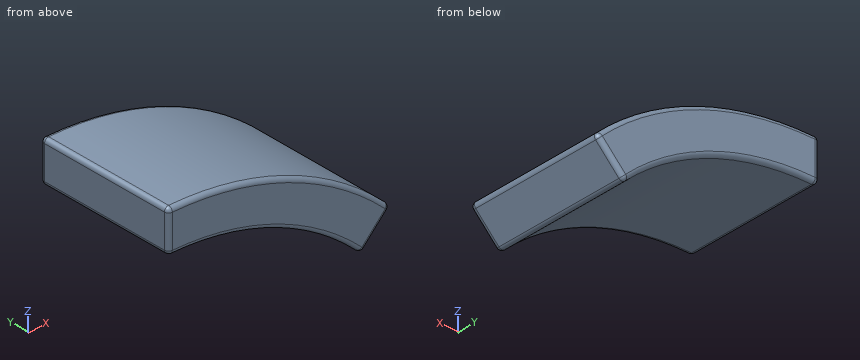
```python
from build123d import *

# Parameters (mm, degrees)
BOSS_EXTRUDE1_DEPTH = 10
FILLET1_R           = 0.3


with BuildPart() as part:
    # Sketch1 → Boss-Extrude1 (new body)
    with BuildSketch(Plane(origin=(0, 0, 0), x_dir=(1, 0, 0), z_dir=(0, 1, 0))):
        with BuildLine():
            Line((14.142135624, -14.142135624), (16.263455967, -16.263455967))
            ThreePointArc((16.263455967, -16.263455967), (8.801718944, -21.249229248), (0, -23))
            Line((0, -23), (0, -20))
            ThreePointArc((0, -20), (7.653668647, -18.47759065), (14.142135624, -14.142135624))
        make_face()
    extrude(amount=BOSS_EXTRUDE1_DEPTH)

    # Fillet1
    fillet1_edges = [part.edges().sort_by_distance(p)[0] for p in [
        (8.801718944, 10, 21.249229248),
        (15.202795796, 10, 15.202795796),
        (7.653668647, 10, 18.47759065),
        (15.202795796, 0, 15.202795796),
        (8.801718944, 0, 21.249229248),
        (0, 0, 21.5),
        (7.653668647, 0, 18.47759065),
        (0, 10, 21.5),
        (14.142135624, 5, 14.142135624),
        (16.263455967, 5, 16.263455967),
        (0, 5, 23),
        (0, 5, 20),
    ]]
    fillet(fillet1_edges, radius=FILLET1_R)


solid = part.part
```
Geometry: final body of the model. Coordinates: model frame, mm. Coordinates: 2 decimals unless noted, no trailing zeros. Order: outer loops, then holes, each group sorted by start corner. A loop starts at its lowest first (then second) coordinate and runs counter-clockwise, first axis right, second up.
Item 1: Material intervals for line 1 along Z through (x, y) = (14.5, 8); line 2 along X through (y, z) = (5.5, 21.25); line 3 along Z through (x, y) = (1, 2.5), sorted ascending.
Answer:
line 1: z = 14.5 to 17.85
line 2: x = 0 to 8.8
line 3: z = 19.97 to 22.98
Item 2: Contact query for flat-ended pins moving along their axis: P1, Ø4, axis at x = 10.5, y = 1, coming from the -Z side; P2, Ø5, axis at x = 11.5, y = 4.5, coming from the -Z side. Output: stop coordinate, or through.
Answer:
P1: stops at z = 15.61
P2: stops at z = 14.3
Item 3: Section query A-A (y = 6.75). Output: boundary loops of the cut face in (x, z).
Answer:
outline: (0, 20.3) arc R0.3 ccw to (0.3, 20) arc R20 cw to (13.93, 14.35) arc R0.3 ccw to (14.35, 14.35) - (16.05, 16.05) arc R0.3 ccw to (16.05, 16.48) arc R23 ccw to (0.3, 23) arc R0.3 ccw to (0, 22.7) - close
